```python
from build123d import *

# Parameters (mm, degrees)
SKETCH1_W           = 80
SKETCH1_H           = 36
BOSS_EXTRUDE1_DEPTH = 5
SKETCH2_W           = 71
SKETCH2_H           = 23.8
BOSS_EXTRUDE2_DEPTH = 2
CUT_EXTRUDE1_REACH  = 345.946
SKETCH3_R           = 0.75


with BuildPart() as part:
    # Sketch1 → Boss-Extrude1 (new body)
    with BuildSketch(Plane.XY):
        with Locations((298.531964754, 42.3820547)):
            Rectangle(SKETCH1_W, SKETCH1_H)
    extrude(amount=BOSS_EXTRUDE1_DEPTH)

    # Sketch2 → Boss-Extrude2 (add)
    with BuildSketch(Plane(origin=(0, 0, 0), x_dir=(-1, 0, 0), z_dir=(0, 0, -1))):
        with Locations((-298.601806293, 42.312213161)):
            Rectangle(SKETCH2_W, SKETCH2_H)
    extrude(amount=BOSS_EXTRUDE2_DEPTH)

    # Sketch3 → Cut-Extrude1 (cut, up to next)
    with BuildSketch(Plane.XY.offset(5), mode=Mode.PRIVATE) as cut_extrude1_sk1:
        with Locations((261.031964754, 25.5070547)):
            Circle(SKETCH3_R)
    cut_extrude1_tool1 = extrude(cut_extrude1_sk1.sketch, amount=-CUT_EXTRUDE1_REACH, mode=Mode.PRIVATE) & part.part
    # Sketch3 → Cut-Extrude1 (cut, up to next)
    with BuildSketch(Plane.XY.offset(5), mode=Mode.PRIVATE) as cut_extrude1_sk2:
        with Locations((336.031964754, 25.5070547)):
            Circle(SKETCH3_R)
    cut_extrude1_tool2 = extrude(cut_extrude1_sk2.sketch, amount=-CUT_EXTRUDE1_REACH, mode=Mode.PRIVATE) & part.part
    # Sketch3 → Cut-Extrude1 (cut, up to next)
    with BuildSketch(Plane.XY.offset(5), mode=Mode.PRIVATE) as cut_extrude1_sk3:
        with Locations((336.031964754, 56.5070547)):
            Circle(SKETCH3_R)
    cut_extrude1_tool3 = extrude(cut_extrude1_sk3.sketch, amount=-CUT_EXTRUDE1_REACH, mode=Mode.PRIVATE) & part.part
    # Sketch3 → Cut-Extrude1 (cut, up to next)
    with BuildSketch(Plane.XY.offset(5), mode=Mode.PRIVATE) as cut_extrude1_sk4:
        with Locations((261.031964754, 56.5070547)):
            Circle(SKETCH3_R)
    cut_extrude1_tool4 = extrude(cut_extrude1_sk4.sketch, amount=-CUT_EXTRUDE1_REACH, mode=Mode.PRIVATE) & part.part
    add(cut_extrude1_tool1.solids().sort_by_distance((261.031965, 25.507055, 5))[0], mode=Mode.SUBTRACT)
    add(cut_extrude1_tool2.solids().sort_by_distance((336.031965, 25.507055, 5))[0], mode=Mode.SUBTRACT)
    add(cut_extrude1_tool3.solids().sort_by_distance((336.031965, 56.507055, 5))[0], mode=Mode.SUBTRACT)
    add(cut_extrude1_tool4.solids().sort_by_distance((261.031965, 56.507055, 5))[0], mode=Mode.SUBTRACT)


solid = part.part
```
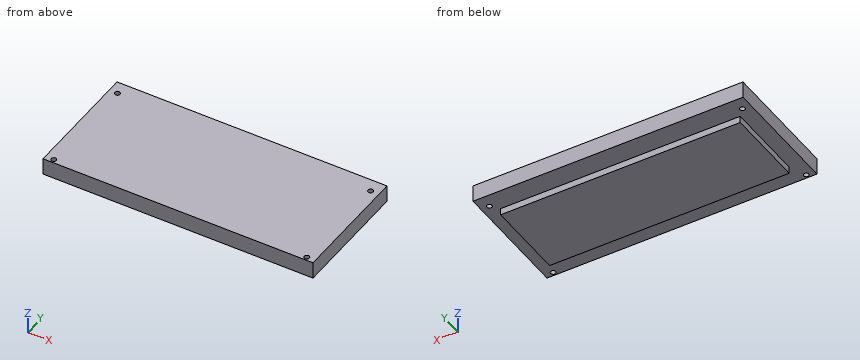
Design review of the part built by this model. Coordinates are the model's own, in mm. Round coordinates to 2 decimals unless told otherwise and drop trailing zeros. Write each loop counter-clockwise with the first axis right and the second up, starting at its lowest first coordinate (ties: lowest second). Pieces come first, ordered by that corner, then holes. Notation, with made-up numbers: (66.25, 45.25) -> (116.25, 45.25) arc R23 cw to (116.25, 56.25) -> close; hole circle Ø9 at (7, 23). An arc over 180 degrees is marked (long way). Answer in a Markdown table with one row per item.
Q1. Take a section at C-C, the plane z = -1. State the section outline as (x, y) points.
The answers:
| item | result |
|---|---|
| outline | (263.1, 30.41) -> (334.1, 30.41) -> (334.1, 54.21) -> (263.1, 54.21) -> close |
Q2. Take a section at D-D, the plane y = 58. State the section outline as (x, z) points, then the cut area to 3 significant figures.
The answers:
| item | result |
|---|---|
| outline | (258.53, 0) -> (338.53, 0) -> (338.53, 5) -> (258.53, 5) -> close |
| area | 400 mm² |
Q3. To check wall thickness, follow L1, parallel to Z at x = 324, y = 56; L2, parallel to Y at x = 275.5, z = -0.25; L3, parallel to X at y = 44, z = -1. State the ranges of each line that lie inside material, in increasing order. Write a range as [from, to].
The answers:
| item | result |
|---|---|
| L1 | [0, 5] |
| L2 | [30.41, 54.21] |
| L3 | [263.1, 334.1] |
Q4. Clearance check with flat-ended pins moving along their axes: pin 1 Ø0.6 at (x, z) = (311.5, -0.5) entering from +Y; pin 2 Ø2 at (x, y) = (336.03, 25.51) entering from -Z. State where each tip first meets the part, or that it passes through.
The answers:
| item | result |
|---|---|
| pin 1 | y = 54.21 |
| pin 2 | z = 0 |
Q5. Take a section at A-A, the plane y = 53.5. State the section outline as (x, z) points.
The answers:
| item | result |
|---|---|
| outline | (258.53, 0) -> (263.1, 0) -> (263.1, -2) -> (334.1, -2) -> (334.1, 0) -> (338.53, 0) -> (338.53, 5) -> (258.53, 5) -> close |
Q6. Take a section at B-B, the plane x = 296.5. State the section outline as (y, z) points, then the cut area to 3 significant figures.
The answers:
| item | result |
|---|---|
| outline | (24.38, 0) -> (30.41, 0) -> (30.41, -2) -> (54.21, -2) -> (54.21, 0) -> (60.38, 0) -> (60.38, 5) -> (24.38, 5) -> close |
| area | 228 mm² |
